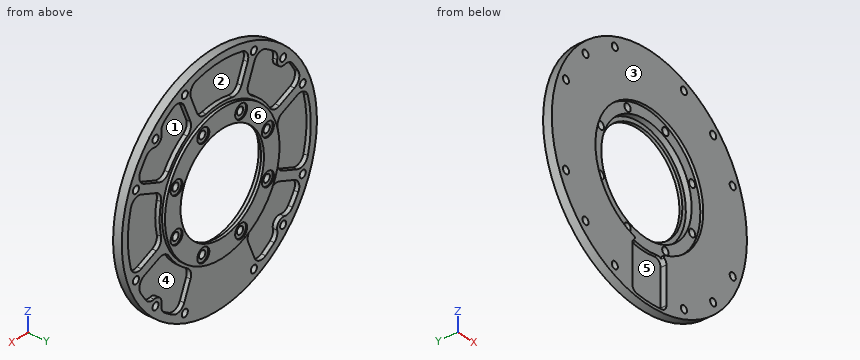
from build123d import *

# Parameters (mm, degrees)
SKETCH_2_R               = 40
EXTRUDE_1_DEPTH          = 4
SKETCH_3_R               = 23.5
EXTRUDE_2_DEPTH          = 1
SKETCH_4_R               = 17.1
CUT_EXTRUDE_1_DEPTH      = 57.789083458
SKETCH_5_R               = 33.5
CUT_EXTRUDE_2_DEPTH      = 1
SKETCH_6_R               = 22.1
CUT_EXTRUDE_3_DEPTH      = 1
SKETCH_7_R               = 18.52
CUT_EXTRUDE_4_DEPTH      = 2
HOLE_WIZARD_M3_1_D       = 2.5
CUT_EXTRUDE_5_DEPTH      = 1.5
PATTERN_CIRCULAR_1_COUNT = 2
PATTERN_CIRCULAR_1_ANGLE = 90
F_1_THE_OTHER_WAY_COUNT  = 2
F_1_THE_OTHER_WAY_ANGLE  = 90
CUT_EXTRUDE_6_DEPTH      = 1.5
PATTERN_CIRCULAR_2_COUNT = 4
CUT_EXTRUDE_7_DEPTH      = 3
FILLET_1_DEPTH           = 2
SKETCH_17_R              = 2.45
CUT_EXTRUDE_8_DEPTH      = 0.4
SKETCH_18_R              = 1.3
CUT_EXTRUDE_9_DEPTH      = 57.755264073
PATTERN_CIRCULAR_3_COUNT = 8
SKETCH_19_W              = 100
SKETCH_19_H              = 100
CUT_EXTRUDE_11_DEPTH     = 1


with BuildPart() as part:
    # 草图2 → 凸台-拉伸1 (new body)
    with BuildSketch(Plane(origin=(0, 0, 0), x_dir=(1, 0, 0), z_dir=(0, 1, 0))):
        with Locations(Location((0, 0, 0), (0, 0, 270))):
            Circle(SKETCH_2_R)
    extrude(amount=EXTRUDE_1_DEPTH)

    # 草图3 → 凸台-拉伸2 (add)
    with BuildSketch(Plane(origin=(0, 4, 0), x_dir=(1, 0, 0), z_dir=(0, 1, 0))):
        with Locations(Location((0, 0, 0), (0, 0, 270))):
            Circle(SKETCH_3_R)
    extrude(amount=EXTRUDE_2_DEPTH)

    # 草图4 → 切除-拉伸1 (cut, through all)
    with BuildSketch(Plane(origin=(0, 5, 0), x_dir=(1, 0, 0), z_dir=(0, 1, 0))):
        with Locations(Location((0, 0, 0), (0, 0, 270))):
            Circle(SKETCH_4_R)
    extrude(amount=-CUT_EXTRUDE_1_DEPTH, mode=Mode.SUBTRACT)

    # 草图5 → 切除-拉伸2 (cut)
    with BuildSketch(Plane.XZ):
        with Locations(Location((0, 0, 0), (0, 0, 270))):
            Circle(SKETCH_5_R)
    extrude(amount=-CUT_EXTRUDE_2_DEPTH, mode=Mode.SUBTRACT)

    # 草图6 → 切除-拉伸3 (cut)
    with BuildSketch(Plane.XZ.offset(-1)):
        with Locations(Location((0, 0, 0), (0, 0, 270))):
            Circle(SKETCH_6_R)
    extrude(amount=-CUT_EXTRUDE_3_DEPTH, mode=Mode.SUBTRACT)

    # 草图7 → 切除-拉伸4 (cut)
    with BuildSketch(Plane.XZ.offset(-2)):
        with Locations(Location((0, 0, 0), (0, 0, 270))):
            Circle(SKETCH_7_R)
    extrude(amount=-CUT_EXTRUDE_4_DEPTH, mode=Mode.SUBTRACT)

    # M3 螺纹孔1 (through all)
    with Locations(Plane(origin=(0, 4, 0), x_dir=(1, 0, 0), z_dir=(0, 1, 0))):
        with Locations((26.162950904, 26.162950904), (-26.162950904, -26.162950904), (-26.162950904, 26.162950904), (26.162950904, -26.162950904), (-14.159286998, 34.183542703), (14.159286998, 34.183542703), (34.183542703, 14.159286998), (34.183542703, -14.159286998), (14.159286998, -34.183542703), (-14.159286998, -34.183542703), (-34.183542703, -14.159286998), (-34.183542703, 14.159286998)):
            Hole(HOLE_WIZARD_M3_1_D / 2)

    # 草图11 → 切除-拉伸5 (cut)
    with BuildSketch(Plane(origin=(0, 4, 0), x_dir=(1, 0, 0), z_dir=(0, 1, 0))):
        with BuildLine():
            Line((-9.060807589, -25.794413462), (-11.616409968, -31.964183385))
            ThreePointArc((-11.616409968, -31.964183385), (-11.525331247, -34.613498711), (-9.46792507, -36.285098799))
            ThreePointArc((-9.46792507, -36.285098799), (0, -37.5), (9.46792507, -36.285098799))
            ThreePointArc((9.46792507, -36.285098799), (11.525331247, -34.613498711), (11.616409968, -31.964183385))
            Line((11.616409968, -31.964183385), (9.060807589, -25.794413462))
            ThreePointArc((9.060807589, -25.794413462), (7.576262006, -24.177592013), (5.39919244, -23.897671874))
            ThreePointArc((5.39919244, -23.897671874), (0, -24.5), (-5.39919244, -23.897671874))
            ThreePointArc((-5.39919244, -23.897671874), (-7.576262006, -24.177592013), (-9.060807589, -25.794413462))
        make_face()
    cut_extrude_5 = extrude(amount=-CUT_EXTRUDE_5_DEPTH, mode=Mode.SUBTRACT)

    # 阵列(圆周)1: 切除-拉伸5 ×2 about axis
    pattern_circular_1_axis = Axis((0, 0, 0), (0, 1, 0))
    for i in range(1, PATTERN_CIRCULAR_1_COUNT):
        add(cut_extrude_5.rotate(pattern_circular_1_axis, i * PATTERN_CIRCULAR_1_ANGLE / (PATTERN_CIRCULAR_1_COUNT - 1)), mode=Mode.SUBTRACT)

    # 1 the other way: 切除-拉伸5 ×2 about axis
    f_1_the_other_way_axis = Axis((0, 0, 0), (0, -1, 0))
    for i in range(1, F_1_THE_OTHER_WAY_COUNT):
        add(cut_extrude_5.rotate(f_1_the_other_way_axis, i * F_1_THE_OTHER_WAY_ANGLE / (F_1_THE_OTHER_WAY_COUNT - 1)), mode=Mode.SUBTRACT)

    # 草图15 → 切除-拉伸6 (cut)
    with BuildSketch(Plane(origin=(0, 4, 0), x_dir=(1, 0, 0), z_dir=(0, 1, 0))):
        with BuildLine():
            Line((-24.646363165, -11.832446186), (-30.816133088, -14.388048565))
            ThreePointArc((-30.816133088, -14.388048565), (-32.625079539, -16.325799779), (-32.352273438, -18.962605396))
            ThreePointArc((-32.352273438, -18.962605396), (-31.217265421, -20.778169786), (-29.980485961, -22.52599524))
            ThreePointArc((-29.980485961, -22.52599524), (-28.524951236, -23.607746352), (-26.715231717, -23.724716727))
            ThreePointArc((-26.715231717, -23.724716727), (-24.395183951, -24.395183951), (-23.724716727, -26.715231717))
            ThreePointArc((-23.724716727, -26.715231717), (-23.607746352, -28.524951236), (-22.52599524, -29.980485961))
            ThreePointArc((-22.52599524, -29.980485961), (-20.778169786, -31.217265421), (-18.962605396, -32.352273438))
            ThreePointArc((-18.962605396, -32.352273438), (-16.325799779, -32.625079539), (-14.388048565, -30.816133088))
            Line((-14.388048565, -30.816133088), (-11.832446186, -24.646363165))
            ThreePointArc((-11.832446186, -24.646363165), (-11.738913025, -22.453365506), (-13.08040025, -20.716011424))
            ThreePointArc((-13.08040025, -20.716011424), (-17.324116139, -17.324116139), (-20.716011424, -13.08040025))
            ThreePointArc((-20.716011424, -13.08040025), (-22.453365506, -11.738913025), (-24.646363165, -11.832446186))
        make_face()
    cut_extrude_6 = extrude(amount=-CUT_EXTRUDE_6_DEPTH, mode=Mode.SUBTRACT)

    # 阵列(圆周)2: 切除-拉伸6 ×4 about axis
    pattern_circular_2_axis = Axis((0, 0, 0), (0, 1, 0))
    for i in range(1, PATTERN_CIRCULAR_2_COUNT):
        add(cut_extrude_6.rotate(pattern_circular_2_axis, i * 360 / PATTERN_CIRCULAR_2_COUNT), mode=Mode.SUBTRACT)

    # 草图16 → 切除-拉伸7 (cut)
    with BuildSketch(Plane.XZ):
        with BuildLine():
            Line((-7, -23.821209037), (-7, -36.485613603))
            ThreePointArc((-7, -36.485613603), (-6.453980705, -37.936250645), (-5.086956522, -38.666818764))
            ThreePointArc((-5.086956522, -38.666818764), (0, -39), (5.086956522, -38.666818764))
            ThreePointArc((5.086956522, -38.666818764), (6.453980705, -37.936250645), (7, -36.485613603))
            Line((7, -36.485613603), (7, -23.821209037))
            ThreePointArc((7, -23.821209037), (6.193547742, -22.11885047), (4.365432099, -21.664556367))
            ThreePointArc((4.365432099, -21.664556367), (0, -22.1), (-4.365432099, -21.664556367))
            ThreePointArc((-4.365432099, -21.664556367), (-6.193547742, -22.11885047), (-7, -23.821209037))
        make_face()
    extrude(amount=-CUT_EXTRUDE_7_DEPTH, mode=Mode.SUBTRACT)

    # 圆角1: read off the stored shape, not the designer's step
    # 圆角1 outline → 圆角1 (cut)
    with BuildSketch(Plane(origin=(0, 0, 0), x_dir=(1, 0, 0), z_dir=(0, 1, 0))):
        with BuildLine():
            ThreePointArc((-4.365432099, 21.664556367), (-5.288780383, 21.676193014), (-6.126015716, 22.06573693))
            ThreePointArc((-6.126015716, 22.06573693), (-5.935396115, 21.57760895), (-6.285184187, 21.187412766))
            ThreePointArc((-6.285184187, 21.187412766), (-5.330649428, 21.447474832), (-4.365432099, 21.664556367))
        make_face()
        with BuildLine():
            ThreePointArc((4.365432099, 21.664556367), (5.330649428, 21.447474832), (6.285184187, 21.187412766))
            ThreePointArc((6.285184187, 21.187412766), (5.935396115, 21.57760895), (6.126015716, 22.06573693))
            ThreePointArc((6.126015716, 22.06573693), (5.288780383, 21.676193014), (4.365432099, 21.664556367))
        make_face()
    extrude(amount=FILLET_1_DEPTH, mode=Mode.SUBTRACT)

    # 草图17 → 切除-拉伸8 (cut)
    with BuildSketch(Plane(origin=(0, 5, 0), x_dir=(1, 0, 0), z_dir=(0, 1, 0))):
        with Locations(Location((7.749339505, -18.708560533, 0), (0, 0, 270))):
            Circle(SKETCH_17_R)
    cut_extrude_8 = extrude(amount=-CUT_EXTRUDE_8_DEPTH, mode=Mode.SUBTRACT)

    # 草图18 → 切除-拉伸9 (cut, through all)
    with BuildSketch(Plane(origin=(0, 4.6, 0), x_dir=(1, 0, 0), z_dir=(0, 1, 0))):
        with Locations(Location((7.749339505, -18.708560533, 0), (0, 0, 270))):
            Circle(SKETCH_18_R)
    cut_extrude_9 = extrude(amount=-CUT_EXTRUDE_9_DEPTH, mode=Mode.SUBTRACT)

    # 阵列(圆周)3: 切除-拉伸8, 切除-拉伸9 ×8 about axis
    pattern_circular_3_axis = Axis((0, 0, 0), (0, 1, 0))
    add([cut_extrude_8.rotate(pattern_circular_3_axis, i * 360 / PATTERN_CIRCULAR_3_COUNT) for i in range(1, PATTERN_CIRCULAR_3_COUNT)], mode=Mode.SUBTRACT)
    add([cut_extrude_9.rotate(pattern_circular_3_axis, i * 360 / PATTERN_CIRCULAR_3_COUNT) for i in range(1, PATTERN_CIRCULAR_3_COUNT)], mode=Mode.SUBTRACT)

    # 草图19 → 切除-拉伸11 (cut)
    with BuildSketch(Plane.XZ):
        Rectangle(SKETCH_19_W, SKETCH_19_H)
    extrude(amount=-CUT_EXTRUDE_11_DEPTH, mode=Mode.SUBTRACT)


solid = part.part
The model under review builds one solid part; all positions refer to its coordinate system, in mm. Face numbers are marked on the shaded views. A direction names the side the tool comes from. Give positions to 0.01 mm unless a question says otherwise; leave off trailing zeros. Loops run counter-clockwise (first coordinate to the right, second up) from the corner with the lowest first, then second, coordinate; pieces in that order, holes last. Notation, with made-up numbers: (58, 21.5) -> (110, 21.5) arc R26 ccw to (110, 36.5) -> close; hole circle Ø7 at (-14, 2.5). An arc over 180 degrees is marked (long way). Put each result on its own line as item: value. Start each with the question number.
1. Mouldability with a two-part tool opening along X and no side actions: class the marked faces 1, 2 and 3 as released by +X, released by -X, zero draft, split by the parting line, or undercut.
2. We need section B-B on z = 0. State the section outline as (x, y) points.
3. Clearance check with flat-ended pins moving along their axes: P1, Ø2, axis at x = 21.5, y = 2, coming from the +Z side; P2, Ø2, axis at y = 1.5, z = -27.5, coming from the -X side; P3, Ø3.5, axis at x = -7.75, z = -18.71, coming from the -Y side; P4, Ø4, axis at x = -8.5, z = 18.5, coming from the +Y side. State where each tip first meets the part, or that it passes through.
4. We need section A-A on x = 0. State the section outline as (y, z) points.
5. We need section C-C on z = -29. State the section outline as (x, y) points.
6. Wall thickness on probe 1 along X at (y, z) = (3.1, 0.5); probe 2 along X at (y, z) = (4.3, 0); probe 3 along Z at (x, y) = (8, 4.3): over which ranges is each line inside the solid? List them lowest first.
7. For the marked faces 4, 5 and 6, list the 3-axis set-ups (+Z, -Z, +X, -X, +Y, -Y) from which the entire face can be reached by the end or side of a thin tool; tool diameter is ignored.
Determined:
1. face 1: undercut
1. face 2: undercut
1. face 3: zero draft
2. outline: (-40, 1) -> (-22.1, 1) -> (-22.1, 2) -> (-18.52, 2) -> (-18.52, 4) -> (-17.1, 4) -> (-17.1, 5) -> (-23.5, 5) -> (-23.5, 4) -> (-24.5, 4) -> (-24.5, 2.5) -> (-37.5, 2.5) -> (-37.5, 4) -> (-40, 4) -> close; (17.1, 4) -> (18.52, 4) -> (18.52, 2) -> (22.1, 2) -> (22.1, 1) -> (40, 1) -> (40, 4) -> (37.5, 4) -> (37.5, 2.5) -> (24.5, 2.5) -> (24.5, 4) -> (23.5, 4) -> (23.5, 5) -> (17.1, 5) -> close
3. P1: z = 34.35
3. P2: x = -29.96
3. P3: y = 2
3. P4: y = 5
4. outline: (1, -40) -> (4, -40) -> (4, -23.5) -> (5, -23.5) -> (5, -17.1) -> (4, -17.1) -> (4, -18.52) -> (2, -18.52) -> (2, -22.1) -> (3, -22.1) -> (3, -39) -> (1, -39) -> close; (1, 22.1) -> (2, 22.1) -> (2, 18.52) -> (4, 18.52) -> (4, 17.1) -> (5, 17.1) -> (5, 23.5) -> (4, 23.5) -> (4, 24.5) -> (2.5, 24.5) -> (2.5, 37.5) -> (4, 37.5) -> (4, 40) -> (1, 40) -> close
5. outline: (-27.55, 1) -> (-7, 1) -> (-7, 3) -> (7, 3) -> (7, 1) -> (27.55, 1) -> (27.55, 4) -> (23.39, 4) -> (23.39, 2.5) -> (13.64, 2.5) -> (13.64, 4) -> (-13.64, 4) -> (-13.64, 2.5) -> (-23.39, 2.5) -> (-23.39, 4) -> (-27.55, 4) -> close
6. probe 1: -40 to -37.5, -24.49 to -18.51, 18.51 to 24.49, 37.5 to 40
6. probe 2: -23.5 to -17.1, 17.1 to 23.5
6. probe 3: -22.1 to -19.98, -17.43 to -15.11, 15.11 to 17.43, 19.98 to 22.1
7. face 4: +Y
7. face 5: -Y
7. face 6: +Z, -Z, +X, -X, +Y
